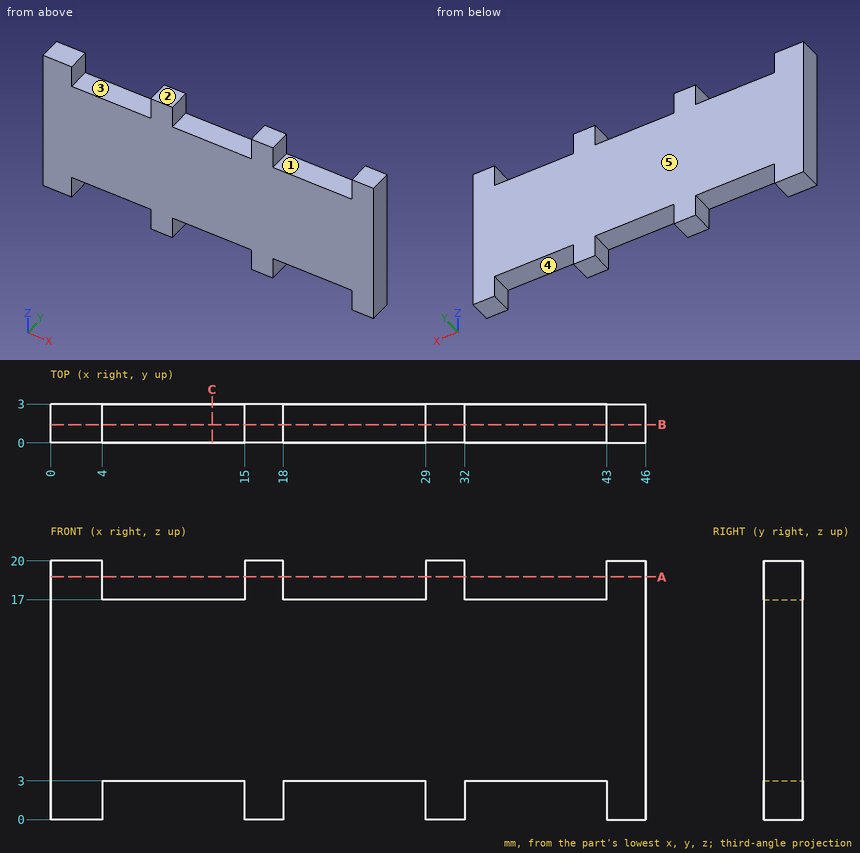
Geometry: see drawing. Coordinates: mm, zero at the bounding-box minimum. A direction names the side the tool comes from. Round coordinates to 2 decimals unless told otherwise and drop trailing zeros. Write each loop counter-clockwise with the first axis right and the second up, starting at its lowest first coordinate (ties: lowest second). Pieces come first, ordered by that corner, then holes. Notation, with made-up numbers: M -21,49.25 L -4,49.25 A10 cw -4,65.25 Z; hole C 89.25,-8 d3. An arc over 180 degrees is marked long. Answer as a JSON object with one key per item and string values. Group by question number.
(1) Section query A-A on z = 18.75. Output: boundary loops of the cut face in (x, y), then the cut area to 3 significant figures.
(2) First-contact query: pin 1 (1.5 mm diameter, centred on x = 22.5, y = 1, fed in from +Z); pin 2 (1.5 mm diameter, centred on x = 24, y = 1, fed in from -Z). Flat tips, straight axial feed; report the tip coordinate or a pass-through.
(3) Section query C-C on x = 12.5. Output: boundary loops of the cut face in (y, z).
(4) Reachability of the marked faces 3, 4 and 5 from +Z, -Z, +X, -X, +Y, -Y: full face, straight path, thin tool, end or side. Return the list, or none.
(5) Mould query, pull axis X, two halves, no side actions, for the marked faces 1 and 2. Classes: +X half, -X half, draft (parallel to the pull), parting line (faces both ways), or undercut.
(6) Ray query, line 1 (X direction, y = 2.15, z = 2.75); line 2 (Z direction, x = 28, y = 0.45). Return the intervals inside material, ascending. Write a range as [from, to].
(7) Section query B-B on y = 1.4. Output: boundary loops of the cut face in (x, z).
Computed values:
{
 "1": {"outline": "M 0,0 L 4,0 L 4,3 L 0,3 Z; M 15,0 L 18,0 L 18,3 L 15,3 Z; M 29,0 L 32,0 L 32,3 L 29,3 Z; M 43,0 L 46,0 L 46,3 L 43,3 Z", "area": "39.0 mm^2"},
 "2": {"pin 1": "z = 17", "pin 2": "z = 3"},
 "3": {"outline": "M 0,3 L 3,3 L 3,17 L 0,17 Z"},
 "4": {"face 3": "+Z, +Y, -Y", "face 4": "-Z, +Y, -Y", "face 5": "+Z, -Z, +X, -X, +Y"},
 "5": {"face 1": "undercut", "face 2": "draft"},
 "6": {"line 1": "[0, 4], [15, 18], [29, 32], [43, 46]", "line 2": "[3, 17]"},
 "7": {"outline": "M 0,0 L 4,0 L 4,3 L 15,3 L 15,0 L 18,0 L 18,3 L 29,3 L 29,0 L 32,0 L 32,3 L 43,3 L 43,0 L 46,0 L 46,20 L 43,20 L 43,17 L 32,17 L 32,20 L 29,20 L 29,17 L 18,17 L 18,20 L 15,20 L 15,17 L 4,17 L 4,20 L 0,20 Z"}
}
